Check sheet for the modelled part. Datum: model origin and axes. Units: mm. Face numbers are marked on the shaded views. Round coordinates to 2 decimals unless told otherwise and drop trailing zeros. Loops run counter-clockwise (first coordinate to the right, second up) from the corner with the lowest first, then second, coordinate; pieces in that order, holes last. Notation, with made-up numbers: (-39, 19.5) -> (-28, 19.5) arc R25 ccw to (-28, 57.5) -> close; hole circle Ø2 at (-36, -17.5). An arc over 180 degrees is marked (long way). Return JSON: item names as keys, results as strings.
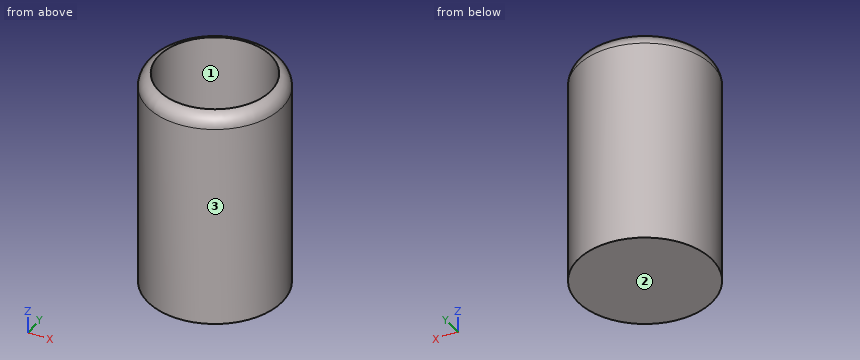
from build123d import *

# Parameters (mm, degrees)
F0_R     = 38.1
F1_DEPTH = 123.825
F2_T     = -6.35


# Not quite as in the source:
# - a fillet or chamfer that OpenCascade refuses, or shapes differently, is made with other operations: its cross-section is extruded or revolved along the edge and cut away or added


with BuildPart() as f1:
    # F0 (on Top) → F1 (new body)
    with BuildSketch(Plane.XY):
        Circle(F0_R)
    extrude(amount=F1_DEPTH)

    # F2
    f2_openings = [f1.faces().sort_by_distance(p)[0] for p in [
        (0, 0, 123.825),
    ]]
    offset(amount=F2_T, openings=f2_openings)

    # F3: fillet of radius 7.971733183 on 1 edges, made by hand

    # F3_s1 → F3_t2 (revolve, cut)
    with BuildSketch(Plane.XZ):
        with BuildLine():
            ThreePointArc((38.1, 116.019968839), (36.3119774413, 121.0508984605), (31.75, 123.825))
            Line((31.75, 123.825), (38.1, 123.825))
            Line((38.1, 123.825), (38.1, 116.019968839))
        make_face()
    revolve(axis=Axis((0, 0, 123.825), (0, 0, 1)), mode=Mode.SUBTRACT)


solid = f1.part
Q1. Go/stop test with flat-tipped pins: pin 1 (6 mm diameter, centred on x = -15.5, y = -29.5, fed in from +Z) (3 decimals); pin 2 (1.5 mm diameter, centred on x = 4.5, z = 81, fed in from -Y) (3 decimals); pin 3 (6 mm diameter, centred on x = 19, z = 28.5, fed in from +Y); pin 4 (2 mm diameter, centred on x = 30, y = -3.5, fed in from +Z). Record where each tip stops, or that it passes through.
Results list:
{"pin 1": "z = 123.825", "pin 2": "y = -37.915", "pin 3": "y = 34.58", "pin 4": "z = 6.35"}
Q2. Section check A-A (x = 0). Record the boundary of the cut face in (y, z) (3 decimals).
Results list:
{"outline": "(-38.1, 0) -> (38.1, 0) -> (38.1, 116.02) arc R7.972 ccw to (31.75, 123.825) -> (31.75, 6.35) -> (-31.75, 6.35) -> (-31.75, 123.825) arc R7.972 ccw to (-38.1, 116.02) -> close"}
Q3. Draft check along X on the marked faces 1, 2 and 3. Enter one of: released by +X, released by -X, zero draft, split by the parting line, or undercut.
Results list:
{"face 1": "undercut", "face 2": "zero draft", "face 3": "split by the parting line"}
Q4. Material ranges on line 1 (Y direction, x = 0, z = 79); line 2 (Z direction, x = -12, y = -15.5); line 3 (Z direction, x = 29.5, y = -12), recorded low to high.
Results list:
{"line 1": "-38.1 to -31.75, 31.75 to 38.1", "line 2": "0 to 6.35", "line 3": "0 to 123.8"}
Q5. Section check B-B (z = 102). Record the boundary of the cut face in (x, y), then the cut area to 3 significant figures.
Results list:
{"outline": "circle Ø76.2 at (0, 0); hole circle Ø63.5 at (0, 0)", "area": "1,390 mm^2"}
